Model file for the job. Use its own axes, mm. Face numbers are marked on the shaded views. Round coordinates to 2 decimals unless told otherwise and drop trailing zeros. Order: outer loops, then holes, each group sorted by start corner. A loop starts at its lowest first (then second) coordinate and runs counter-clockwise, first axis right, second up. Notation, with made-up numbers: (14, 41.5) -> (62, 41.5) arc R19 cw to (62, 57.5) -> close; hole circle Ø11 at (53, 43.25). An arc over 180 degrees is marked (long way). Answer as CSV lines item,"result".
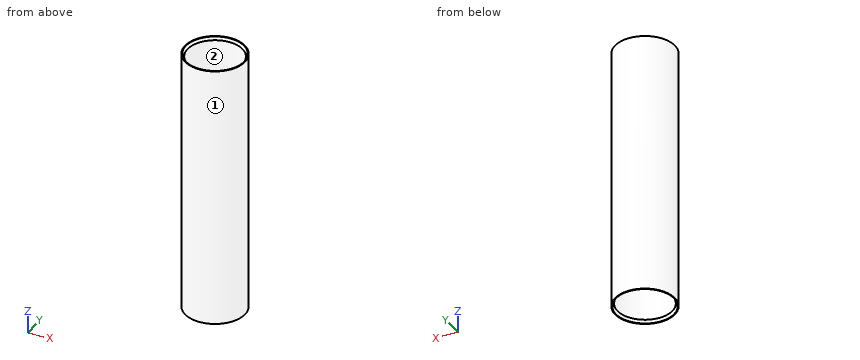
```python
from build123d import *

# Parameters (mm, degrees)
F0_W     = 21
F0_H     = 185
F2_R     = 19.25
F3_DEPTH = 185.001
F4_SIZE2 = 1.1547005384
F4_SIZE  = 2


with BuildPart() as f1:
    # F0 (on Front) → F1 (revolve)
    with BuildSketch(Plane.XZ):
        Rectangle(F0_W, F0_H)
    revolve(axis=Axis((-10.5, 0, 0), (0, 0, 1)))

    # F2 (on face) → F3 (cut, through all)
    with BuildSketch(Plane.XY.offset(92.5)):
        with Locations((-10.5, 0)):
            Circle(F2_R)
    extrude(amount=-F3_DEPTH, mode=Mode.SUBTRACT)

    # F4
    f4_edges = [f1.edges().sort_by_distance(p)[0] for p in [
        (-29.75, 0, 92.5),
        (-29.75, 0, -92.5),
    ]]
    f4_side = f1.faces().sort_by_distance((-29.75, 0, 0))[0]
    chamfer(f4_edges, length=F4_SIZE, length2=F4_SIZE2, reference=f4_side)


solid = f1.part
```
Q1. Mould opens along X. For the marked faces 1 and 2 say: +X half, -X half, draft (parallel to the pull), parting line (faces both ways), or undercut.
Checks:
face 1,"parting line"
face 2,"undercut"
Q2. Saw through at B-B (y = 0). Write the cut outline in (x, z).
Checks:
outline,"(-31.5, -92.5) -> (-30.9, -92.5) -> (-29.75, -90.5) -> (-29.75, 90.5) -> (-30.9, 92.5) -> (-31.5, 92.5) -> close; (8.75, -90.5) -> (9.9, -92.5) -> (10.5, -92.5) -> (10.5, 92.5) -> (9.9, 92.5) -> (8.75, 90.5) -> close"
Q3. Saw through at A-A (x = -10.5). Write the cut outline in (y, z), plus the area to 3 significant figures.
Checks:
outline,"(-21, -92.5) -> (-20.4, -92.5) -> (-19.25, -90.5) -> (-19.25, 90.5) -> (-20.4, 92.5) -> (-21, 92.5) -> close; (19.25, -90.5) -> (20.4, -92.5) -> (21, -92.5) -> (21, 92.5) -> (20.4, 92.5) -> (19.25, 90.5) -> close"
area,"643 mm²"
Q4. Saw through at C-C (z = 10). Write the cut outline in (x, y).
Checks:
outline,"circle Ø42 at (-10.5, 0); hole circle Ø38.5 at (-10.5, 0)"
Q5. Wall check: L1, parallel to Y at x = -10, z = -36; L2, parallel to X at y = -0.5, z = 5.5; L3, parallel to X at y = -17, z = -66. Give the ranges that are in metal, low to high. Write a range as [from, to].
Checks:
L1,"[-20.99, -19.24], [19.24, 20.99]"
L2,"[-31.49, -29.74], [8.74, 10.49]"
L3,"[-22.83, -19.53], [-1.47, 1.83]"
Q6. Flat gauge pins, fed straight in: pin 1 (2 mm diameter, centred on x = -14.5, z = 62.5, fed in from -Y); pin 2 (3 mm diameter, centred on x = -7.5, z = 44, fed in from -Y); pin 3 (10 mm diameter, centred on x = 5, y = -5.5, fed in from -Z); pin 4 (5 mm diameter, centred on x = -2, y = 13, fed in from +Z). Where does each tip first touch, or does it go through?
Checks:
pin 1,"y = -20.78"
pin 2,"y = -20.95"
pin 3,"z = -92.5"
pin 4,"through"
